from build123d import *

# Parameters (mm, degrees)
CUT_EXTRUDE1_DEPTH = 3.048
SKETCH5_R          = 2.749630657
CUT_EXTRUDE2_DEPTH = 3.048
CUT_EXTRUDE2_DRAFT = -45
CHAMFER1_SIZE      = 0.47625


with BuildPart() as part:
    # Sketch3 → Revolve1 (revolve)
    with BuildSketch(Plane(origin=(0, 0, 0), x_dir=(0, 0, -1), z_dir=(1, 0, 0))):
        Polygon((-47.625, 4.7625), (-47.625, 2.38125), (-44.577, 2.38125), (-44.577, 0), (47.625, 0), (47.625, 2.2225), (46.6725, 3.175), (-41.275, 3.175), (-41.275, 4.7625), align=None)
    revolve(axis=Axis((0, 0, 47.625), (0, 0, -1)))

    # Sketch4 → Cut-Extrude1 (cut)
    with BuildSketch(Plane.XY.offset(47.625)):
        Polygon((0, 2.749630657), (-2.38125, 1.374815329), (-2.38125, -1.374815329), (0, -2.749630657), (2.38125, -1.374815329), (2.38125, 1.374815329), align=None)
    extrude(amount=-CUT_EXTRUDE1_DEPTH, mode=Mode.SUBTRACT)


with BuildPart() as cut_extrude2_tool:
    # Sketch5 → Cut-Extrude2 (with draft: the straight prism first)
    with BuildSketch(Plane.XY.offset(47.625)):
        Circle(SKETCH5_R)
    extrude(amount=-CUT_EXTRUDE2_DEPTH)
    # Cut-Extrude2: the draft: its side faces are tilted about the plane it starts from
    cut_extrude2_sides = [cut_extrude2_tool.faces().sort_by_distance(p)[0] for p in [
        (-2.749630657, 0, 46.101),
    ]]
    draft(cut_extrude2_sides, Plane.XY.offset(47.625), CUT_EXTRUDE2_DRAFT)


with BuildPart() as part_1:
    add(part.part)

    # Cut-Extrude2: cut by cut_extrude2_tool
    add(cut_extrude2_tool.part, mode=Mode.SUBTRACT)

    # Chamfer1
    chamfer1_edges = [part_1.edges().sort_by_distance(p)[0] for p in [
        (0, -4.7625, 47.625),
        (0, -4.7625, 41.275),
    ]]
    chamfer(chamfer1_edges, length=CHAMFER1_SIZE)


solid = part_1.part
Geometry check sheet. Reference: the model listing, model coordinates, mm. A direction names the side the tool comes from. Give positions to 0.01 mm unless a question says otherwise; leave off trailing zeros. Order: outer loops, then holes, each group sorted by start corner. A loop starts at its lowest first (then second) coordinate and runs counter-clockwise, first axis right, second up.
1) Draft check along Y on faces 4 (the flat face through (2.381, 0, 46)), 5 (the cylindrical face through (-2.9, -3.78, 44.49)), 6 (the flat face through (-2, 3, 41.275)). Enter one of: released by +Y, released by -Y, zero draft, split by the parting line, or undercut.
Results are:
face 4: undercut
face 5: split by the parting line
face 6: zero draft
2) Material ranges on probe 1 along Z at (x, y) = (3.75, 1.5) (3 decimals); probe 2 along Y at (x, z) = (0.25, -36); probe 3 along Z at (x, y) = (-1.25, -0.5) (3 decimals), recorded low to high.
Results are:
probe 1: z = 41.275 to 47.625
probe 2: y = -3.17 to 3.17
probe 3: z = -47.625 to 44.577
3) Gauge pin test, flat ends, axial feed: pin 1 (0.8 mm diameter, centred on y = 0.5, z = 46, fed in from +X); pin 2 (5 mm diameter, centred on x = 2.5, z = 34, fed in from +Y) (3 decimals); pin 3 (1.5 mm diameter, centred on y = 2.5, z = -26, fed in from +X); pin 4 (4 mm diameter, centred on x = -0.5, z = 6.5, fed in from -Y) (3 decimals). Record the tip position at first contact, or that the pin passes through.
Results are:
pin 1: stops at x = 4.76
pin 2: stops at y = 3.175
pin 3: stops at x = 2.65
pin 4: stops at y = -3.175
4) Cross-section at A-A (y = 0). Record the boundary of the cut face in (x, z) (1 decimal).
Results are:
outline: (-4.8, 41.8) - (-4.3, 41.3) - (-3.2, 41.3) - (-3.2, -46.7) - (-2.2, -47.6) - (2.2, -47.6) - (3.2, -46.7) - (3.2, 41.3) - (4.3, 41.3) - (4.8, 41.8) - (4.8, 47.1) - (4.3, 47.6) - (2.7, 47.6) - (2.4, 47.3) - (2.4, 44.6) - (-2.4, 44.6) - (-2.4, 47.3) - (-2.7, 47.6) - (-4.3, 47.6) - (-4.8, 47.1) - close
5) Cross-section at B-B (z = -24). Record the boundary of the cut face in (x, y) (3 decimals), then the cut area to 3 significant figures.
Results are:
outline: circle Ø6.35 at (0, 0)
area: 31.7 mm2
6) Tool access check on faces 1 (the cylindrical face through (-3.1, -0.69, -2.08)), 2 (the flat face through (0, 3, 47.625)), 3 (the flat face through (1.21, 2.05, 46.12)). Record the directions out of +Z, -Z, +X, -X, +Y, -Y that give a thin tool (end or side, any length) a straight path to the whole face; none if there is none.
Results are:
face 1: -Z
face 2: +Z, +X, -X, +Y, -Y
face 3: +Z
